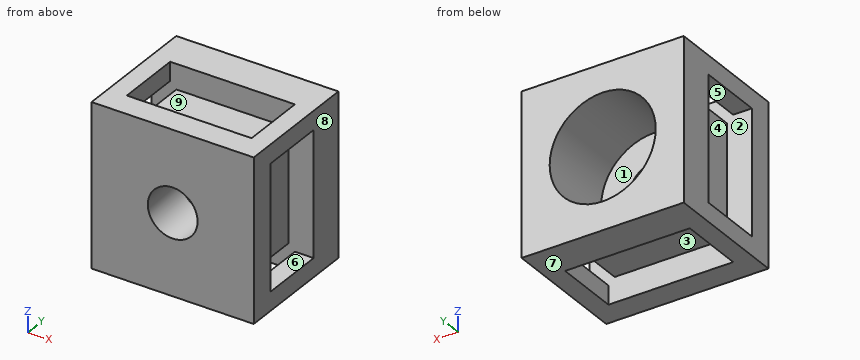
from build123d import *

# Parameters (mm, degrees)
SKETCH2_W                = 26
SKETCH2_H                = 20.5
BOSS_EXTRUDE1_DEPTH      = 26
HAPTUATOR_HOLE_R         = 8.5
HAPTUATORINSERTION_DEPTH = 12.5
SKETCH8_R                = 3.989772047
CLEARANCE_DEPTH          = 43.09809972
CUTOUT_W                 = 20
CUTOUT_H                 = 10.5
CUT_EXTRUDE3_DEPTH       = 4
CIRPATTERN1_COUNT        = 4


with BuildPart() as part:
    # Sketch2 → Boss-Extrude1 (new body)
    with BuildSketch(Plane.XY):
        with Locations((13, 10.25)):
            Rectangle(SKETCH2_W, SKETCH2_H)
    extrude(amount=BOSS_EXTRUDE1_DEPTH)

    # Haptuator Hole → HaptuatorInsertion (cut)
    with BuildSketch(Plane(origin=(0, 20.5, 0), x_dir=(1, 0, 0), z_dir=(0, 1, 0))):
        with Locations(Location((13, -13, 0), (0, 0, 270))):
            Circle(HAPTUATOR_HOLE_R)
    extrude(amount=-HAPTUATORINSERTION_DEPTH, mode=Mode.SUBTRACT)

    # Sketch8 → Clearance (cut, through all)
    with BuildSketch(Plane.XZ):
        with Locations(Location((13, 13, 0), (0, 0, 270))):
            Circle(SKETCH8_R)
    extrude(amount=-CLEARANCE_DEPTH, mode=Mode.SUBTRACT)

    # cutout → Cut-Extrude3 (cut)
    with BuildSketch(Plane.XY.offset(26)):
        with Locations((13, 9.25)):
            Rectangle(CUTOUT_W, CUTOUT_H)
    cut_extrude3 = extrude(amount=-CUT_EXTRUDE3_DEPTH, mode=Mode.SUBTRACT)

    # CirPattern1: Cut-Extrude3 ×4 about axis
    cirpattern1_axis = Axis((13, 0, 13), (0, 1, 0))
    for i in range(1, CIRPATTERN1_COUNT):
        add(cut_extrude3.rotate(cirpattern1_axis, i * 360 / CIRPATTERN1_COUNT), mode=Mode.SUBTRACT)


solid = part.part
The model under review builds one solid part; all positions refer to its coordinate system, in mm. Face numbers are marked on the shaded views. A direction names the side the tool comes from. Give positions to 0.01 mm unless a question says otherwise; leave off trailing zeros. Loops run counter-clockwise (first coordinate to the right, second up) from the corner with the lowest first, then second, coordinate; pieces in that order, holes last. Notation, with made-up numbers: (65.25, 18) -> (85.25, 18) arc R15 ccw to (85.25, 43) -> close; hole circle Ø1 at (34, 49). An arc over 180 degrees is marked (long way). Answer as a JSON object with one key per item and string values. Group by question number.
Q1. Tool access review of the marked faces 1, 2, 3, 4 and 5: name each direction out of +Z, -Z, +X, -X, +Y, -Y from which nothing blocks a thin tool from reaching the whole face with its end or side.
Q2. Take a section at D-D (x = 5.5). Write out the cut boundary in (y, z), plus the area to 3 significant figures.
Q3. Insertion check: pin 1 (1.5 mm diameter, centred on x = 15.5, y = 10.5, fed in from -Z); pin 2 (1 mm diameter, centred on x = 11, z = 12, fed in from +Y); pin 3 (8.5 mm diameter, centred on x = 10.5, z = 16, fed in from +Y); pin 4 (3 mm diameter, centred on y = 11.5, z = 9, fed in from -X). Each pin has a flat end and moves straight along its axis. Give the tip position at first contact, or say it passes through.
Q4. Take a section at A-A (y = 11.5). Write out the cut boundary in (x, z), plus the area to 3 significant figures.
Q5. Wall thickness on line 1 along X through (y, z) = (6.25, 13); line 2 along X through (y, z) = (15, 13); line 3 along Y through (x, z) = (3.25, 17): over which ranges is each line inside the solid? List them lowest first.
Q6. Draft analysis for pull direction Z (two halves, no side actions). For the marked faces 6, 7, 8 and 9, state which applies: pulls with the +Z half, pulls with the -Z half, needs draft (parallel to the pull), parting line crosses it, or undercut.
Q7. Take a section at C-C (z = 13). Write out the cut boundary in (x, y), plus the area to 3 significant figures.
Q8. Take a section at B-B (x = 13). Write out the cut boundary in (y, z).
Answer below:
{
 "1": {"face 1": "+Y", "face 2": "none", "face 3": "-Z, +X, -X", "face 4": "+Z, -Z, -X", "face 5": "+X, -X"},
 "2": {"outline": "(0, 0) -> (4, 0) -> (4, 4) -> (14.5, 4) -> (14.5, 0) -> (20.5, 0) -> (20.5, 9) -> (8, 9) -> (8, 17) -> (20.5, 17) -> (20.5, 26) -> (14.5, 26) -> (14.5, 22) -> (4, 22) -> (4, 26) -> (0, 26) -> close", "area": "349 mm2"},
 "3": {"pin 1": "stops at z = 4", "pin 2": "passes through", "pin 3": "stops at y = 8", "pin 4": "stops at x = 4"},
 "4": {"outline": "(0, 0) -> (3, 0) -> (3, 3) -> (0, 3) -> close; (0, 23) -> (3, 23) -> (3, 26) -> (0, 26) -> close; (4, 4) -> (22, 4) -> (22, 22) -> (4, 22) -> close; (23, 0) -> (26, 0) -> (26, 3) -> (23, 3) -> close; (23, 23) -> (26, 23) -> (26, 26) -> (23, 26) -> close; hole circle Ø17 at (13, 13)", "area": "133 mm2"},
 "5": {"line 1": "x = 4 to 9.01, 16.99 to 22", "line 2": "x = 0 to 4.5, 21.5 to 26", "line 3": "y = 0 to 4, 14.5 to 20.5"},
 "6": {"face 6": "undercut", "face 7": "pulls with the -Z half", "face 8": "needs draft", "face 9": "pulls with the +Z half"},
 "7": {"outline": "(0, 0) -> (9.01, 0) -> (9.01, 8) -> (4.5, 8) -> (4.5, 20.5) -> (0, 20.5) -> (0, 14.5) -> (4, 14.5) -> (4, 4) -> (0, 4) -> close; (16.99, 0) -> (26, 0) -> (26, 4) -> (22, 4) -> (22, 14.5) -> (26, 14.5) -> (26, 20.5) -> (21.5, 20.5) -> (21.5, 8) -> (16.99, 8) -> close", "area": "173 mm2"},
 "8": {"outline": "(0, 0) -> (4, 0) -> (4, 4) -> (14.5, 4) -> (14.5, 0) -> (20.5, 0) -> (20.5, 4.5) -> (8, 4.5) -> (8, 9.01) -> (0, 9.01) -> close; (0, 16.99) -> (8, 16.99) -> (8, 21.5) -> (20.5, 21.5) -> (20.5, 26) -> (14.5, 26) -> (14.5, 22) -> (4, 22) -> (4, 26) -> (0, 26) -> close"}
}
